Here's how the part is built. I have some questions about the finished solid (model axes, mm). Face numbers are marked on the shaded views. Round coordinates to 2 decimals unless told otherwise and drop trailing zeros. Write each loop counter-clockwise with the first axis right and the second up, starting at its lowest first coordinate (ties: lowest second). Pieces come first, ordered by that corner, then holes. Notation, with made-up numbers: M -21.75,56.5 L 12.25,56.5 A16 cw 12.25,74.5 Z; hole C 85.25,-26.5 d8. An arc over 180 degrees is marked long. Write item = value, one per line. Start each with the question number.
(1) Will these pins go through, and if not, where does the flat tip stop? pin 1 Ø8 at (x, z) = (20, 16.5) entering from -Y; pin 2 Ø10 at (y, z) = (4, 17.5) entering from -X (1 decimal); pin 3 Ø2 at (y, z) = (30.5, 5) entering from +X; pin 4 Ø1.5 at (x, y) = (-17, -26) entering from +Z.
(2) If we mould it in two halves opening along X, with no side actions, what happens to the marked faces 1, 2 and 3? For each: released by +X, released by -X, zero draft, split by the parting line, or undercut.
(3) I want a section at A-A (z = 11). List the corners of the cut face in (x, y) for me.
(4) I want a section at B-B (x = -6). Give the number of separate pieces and of enclosed holes in the cut face, and give its area (3 significant figures).
(5) I need wall thicknesses on line 1 along Y through (x, z) = (0, 5.15); line 2 along X through (y, z) = (16.5, 28.5); line 3 along Z through (x, y) = (-34, -22). Which ranges of each line are inside material? Lowest first, please.
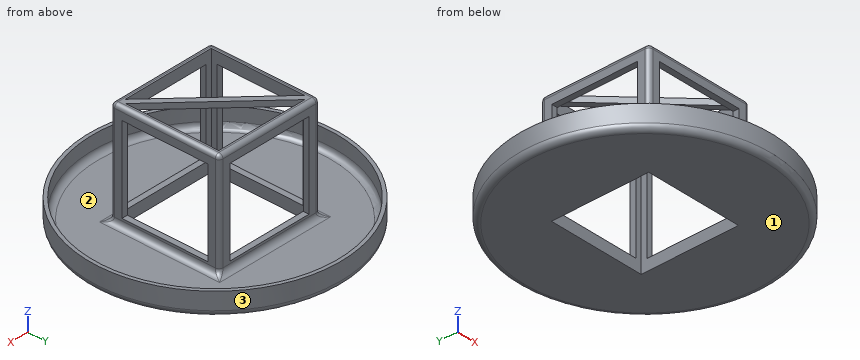
```python
from build123d import *

# Parameters (mm, degrees)
SKETCH001_R          = 44.2
SKETCH001_W          = 34
SKETCH001_H          = 34
PAD_DEPTH            = 1.2
SKETCH002_W          = 38
SKETCH002_H          = 38
SKETCH002_W_2        = 34
SKETCH002_H_2        = 34
PAD001_DEPTH         = 36
SKETCH003_W          = 38
SKETCH003_H          = 38
PAD002_DEPTH         = 2
SKETCH004_W          = 30
SKETCH004_H          = 30
POCKET_DEPTH         = 44.201
POCKET_DEPTH_BACK    = -44.201
SKETCH005_W          = 30
SKETCH005_H          = 30
POCKET001_DEPTH      = 44.201
POCKET001_DEPTH_BACK = -44.201
POCKET002_DEPTH      = 299.329299
POLARPATTERN_COUNT   = 2
SKETCH007_R          = 44.2
SKETCH007_R_2        = 43
PAD003_DEPTH         = 8
FILLET_R             = 2
FILLET001_R          = 2
FILLET002_R          = 1.4


with BuildPart() as part:
    # Sketch001 → Pad (new body)
    with BuildSketch(Plane.XY):
        Circle(SKETCH001_R)
        Rectangle(SKETCH001_W, SKETCH001_H, mode=Mode.SUBTRACT)
    extrude(amount=PAD_DEPTH)

    # Sketch002 → Pad001 (join)
    with BuildSketch(Plane.XY):
        Rectangle(SKETCH002_W, SKETCH002_H)
        Rectangle(SKETCH002_W_2, SKETCH002_H_2, mode=Mode.SUBTRACT)
    extrude(amount=PAD001_DEPTH)

    # Sketch003 (on Plane of DatumPlane) → Pad002 (join)
    with BuildSketch(Plane.XY.offset(36)):
        Rectangle(SKETCH003_W, SKETCH003_H)
    extrude(amount=PAD002_DEPTH)

    # Sketch004 → Pocket (cut, two sides)
    with BuildSketch(Plane.YZ) as pocket_sk:
        with Locations((0, 19)):
            Rectangle(SKETCH004_W, SKETCH004_H)
    extrude(amount=-POCKET_DEPTH, mode=Mode.SUBTRACT)
    extrude(pocket_sk.sketch, amount=-POCKET_DEPTH_BACK, mode=Mode.SUBTRACT)

    # Sketch005 → Pocket001 (cut, two sides)
    with BuildSketch(Plane.XZ) as pocket001_sk:
        with Locations((0, 19)):
            Rectangle(SKETCH005_W, SKETCH005_H)
    extrude(amount=-POCKET001_DEPTH, mode=Mode.SUBTRACT)
    extrude(pocket001_sk.sketch, amount=-POCKET001_DEPTH_BACK, mode=Mode.SUBTRACT)

    # Sketch006 → Pocket002 (cut, through all)
    with BuildSketch(Plane.XY):
        Polygon((-17, 15.585786), (-17, -17), (15.585786, -17), align=None)
    pocket002 = extrude(amount=POCKET002_DEPTH, mode=Mode.SUBTRACT)

    # PolarPattern: Pocket002 ×2 about axis
    polarpattern_axis = Axis((0, 0, 0), (0, 0, 1))
    for i in range(1, POLARPATTERN_COUNT):
        add(pocket002.rotate(polarpattern_axis, i * 360 / POLARPATTERN_COUNT), mode=Mode.SUBTRACT)

    # Sketch007 → Pad003 (join)
    with BuildSketch(Plane.XY):
        Circle(SKETCH007_R)
        Circle(SKETCH007_R_2, mode=Mode.SUBTRACT)
    extrude(amount=PAD003_DEPTH)

    # Fillet
    fillet_edges = [part.edges().sort_by_distance(p)[0] for p in [
        (0, -19, 1.2),
        (-19, 0, 1.2),
        (19, 0, 1.2),
        (0, 19, 1.2),
        (-43, 0, 1.2),
    ]]
    fillet(fillet_edges, radius=FILLET_R)

    # Fillet001
    fillet001_edges = [part.edges().sort_by_distance(p)[0] for p in [
        (-44.2, 0, 0),
    ]]
    fillet(fillet001_edges, radius=FILLET001_R)

    # Fillet002
    fillet002_edges = [part.edges().sort_by_distance(p)[0] for p in [
        (19, 0, 38),
        (0, -19, 38),
        (-19, 0, 38),
        (0, 19, 38),
        (19, 19, 19.6),
        (19, -19, 19.6),
        (-19, -19, 19.6),
        (-19, 19, 19.6),
    ]]
    fillet(fillet002_edges, radius=FILLET002_R)


solid = part.part
```
Returned:
q1.pin_1 = -19
q1.pin_2 = through
q1.pin_3 = 32.91
q1.pin_4 = 1.2
q2.face_1 = zero draft
q2.face_2 = undercut
q2.face_3 = split by the parting line
q3.outline = M -19,-17.6 A1.4 ccw -17.6,-19 L -15,-19 L -15,-17 L -17,-17 L -17,-15 L -19,-15 Z; M -19,15 L -17,15 L -17,17 L -15,17 L -15,19 L -17.6,19 A1.4 ccw -19,17.6 Z; M 15,-19 L 17.6,-19 A1.4 ccw 19,-17.6 L 19,-15 L 17,-15 L 17,-17 L 15,-17 Z; M 15,17 L 17,17 L 17,15 L 19,15 L 19,17.6 A1.4 ccw 17.6,19 L 15,19 Z
q4.separate_pieces = 5
q4.enclosed_holes = 0
q4.area = 115 mm²
q5.line_1 = -44.2 to -43, 43 to 44.2
q5.line_2 = -19 to -17, 17 to 19
q5.line_3 = 0 to 1.2
